from build123d import *

# Parameters (mm, degrees)
BOSS_EXTRUDE1_DEPTH = 39.25
SKETCH4_R           = 13.75
CUT_EXTRUDE1_DEPTH  = 30
SKETCH7_R           = 9.75
SKETCH6_R           = 10.2
SKETCH5_R           = 3.5
CUT_EXTRUDE2_DEPTH  = 15


with BuildPart() as part:
    # Sketch2 → Boss-Extrude1 (new, symmetric)
    with BuildSketch(Plane(origin=(0, 0, 0), x_dir=(0, 0, -1), z_dir=(1, 0, 0))):
        Polygon((-100, -24.35604681), (20, -144.35604681), (20, -24.35604681), align=None)
    extrude(amount=BOSS_EXTRUDE1_DEPTH, both=True)

    # Sketch4 → Cut-Extrude1 (cut)
    with BuildSketch(Plane(origin=(0, -24.35604681, 0), x_dir=(1, 0, 0), z_dir=(0, 1, 0))):
        with Locations(Location((0, 0, 0), (0, 0, 270))):
            Circle(SKETCH4_R)
    extrude(amount=-CUT_EXTRUDE1_DEPTH, mode=Mode.SUBTRACT)

    # Sketch7 → Cut-Loft1 section 0
    with BuildSketch(Plane(origin=(0, -84.35604681, 0), x_dir=(1, 0, 0), z_dir=(0, 1, 0))):
        Circle(SKETCH7_R)
    # Sketch6 → Cut-Loft1 section 1
    with BuildSketch(Plane(origin=(0, -54.35604681, 0), x_dir=(1, 0, 0), z_dir=(0, 1, 0))):
        Circle(SKETCH6_R)
    loft(mode=Mode.SUBTRACT)

    # Sketch5 → Cut-Extrude2 (cut)
    with BuildSketch(Plane(origin=(0, 0, -20), x_dir=(-1, 0, 0), z_dir=(0, 0, -1))):
        with Locations(Location((0, -59.35604681, 0), (0, 0, 90))):
            Circle(SKETCH5_R)
        with Locations(Location((0, -74.35604681, 0), (0, 0, 90))):
            Circle(SKETCH5_R)
    extrude(amount=-CUT_EXTRUDE2_DEPTH, mode=Mode.SUBTRACT)


solid = part.part
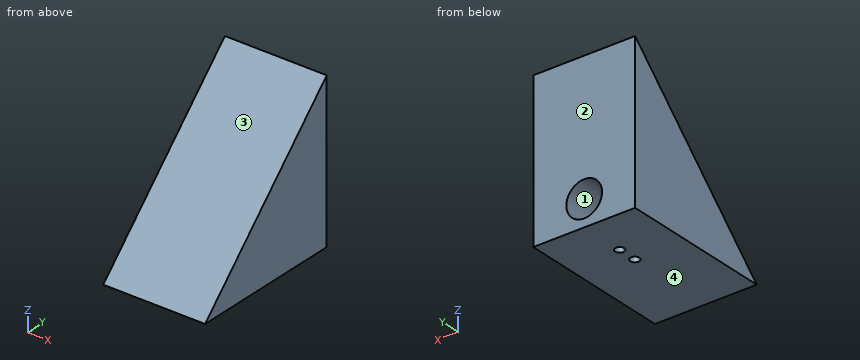
Here's how the part is built. I have some questions about the finished solid (model axes, mm). Face numbers are marked on the shaded views. Coordinates: 2 decimals unless noted, no trailing zeros. Write each loop counter-clockwise with the first axis right and the second up, starting at its lowest first coordinate (ties: lowest second). Pieces come first, ordered by that corner, then holes.
1) If we section it at B-B (z = 65): List the corners of the cut face in (x, y) for me, plus the area to 3 significant figures.
Filled in:
outline: (-39.25, -59.36) - (39.25, -59.36) - (39.25, -24.36) - (-39.25, -24.36) - close
area: 2,750 mm2
2) I'm going to push flat-ended pins straight in: pin 1 (2 mm diameter, centred on x = -11, y = -45.5, fed in from +Z); pin 2 (14 mm diameter, centred on x = -4.5, z = 0.5, fed in from +Y); pin 3 (6.5 mm diameter, centred on x = 0, y = -74.36, fed in from +Z); pin 4 (10 mm diameter, centred on y = -98.5, z = 36, fed in from +X). Where does each tip first touch, or does it pass through?
Filled in:
pin 1: stops at z = 79.86
pin 2: stops at y = -54.36
pin 3: stops at z = 53.25
pin 4: passes through
3) If we section it at D-D (z = 91): List the corners of the cut face in (x, y) for me, plus the area to 4 significant figures.
Filled in:
outline: (-39.25, -33.36) - (39.25, -33.36) - (39.25, -24.36) - (-39.25, -24.36) - close
area: 706.5 mm2
4) Thinking about a two-plate mould opening in Z: for the marked faces 1, 2, 3 and 4, which applies, +Z half, -Z half, draft (parallel to the pull), parting line (faces both ways), or undercut?
Filled in:
face 1: undercut
face 2: draft
face 3: +Z half
face 4: -Z half
5) If we section it at A-A (x = 0): Count the separate pieces of the cut face and the enclosed holes in it, plus the area to 3 significant figures.
Filled in:
separate pieces: 3
enclosed holes: 0
area: 5,640 mm2
6) If I drill on line 1 (Y direction, x = 0, z = -13); line 2 (Y direction, x = 0, z = -14.25); line 3 (Z direction, x = -3.5, y = -61.5), over which ranges is the centre line in solid material (lowest first)?
Filled in:
line 1: y = -137.36 to -77.86, -70.86 to -62.86, -55.86 to -54.36
line 2: y = -138.61 to -77.86, -70.86 to -62.86, -55.86 to -24.36
line 3: z = -20 to -9.47, 9.47 to 62.86
7) If we section it at C-C (x = -28.5): List the corners of the cut face in (y, z) for me.
Filled in:
outline: (-144.36, -20) - (-24.36, -20) - (-24.36, 100) - close
